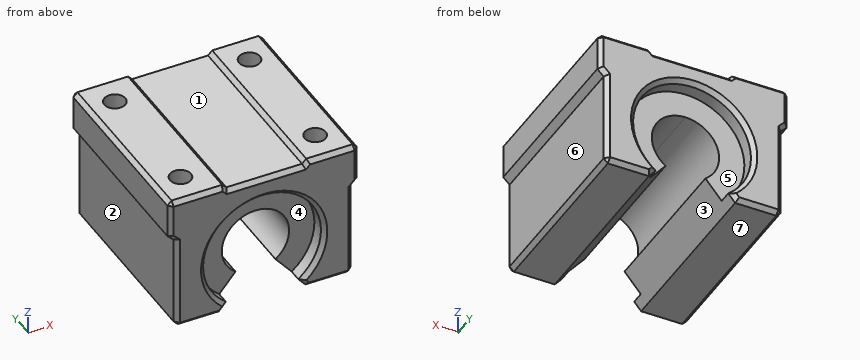
```python
from build123d import *

# Parameters (mm, degrees)
F1_DEPTH = 45
F2_R     = 14
F3_DEPTH = 4
F4_R     = 14
F5_DEPTH = 4
F6_R     = 2.5
F7_DEPTH = 12
F8_SIZE  = 1


with BuildPart() as f1:
    # F0 (on Front) → F1 (new body)
    with BuildSketch(Plane.XZ):
        with BuildLine():
            Line((13, 33), (0, 33))
            Line((0, 33), (0, 24))
            Line((0, 24), (1.5, 22.5))
            Line((1.5, 22.5), (1.5, 0))
            Line((1.5, 0), (12.250585, 0))
            Line((12.250585, 0), (17.754591, 6.559418))
            ThreePointArc((17.754591, 6.559418), (14.899847, 15.497533), (22.5, 21))
            ThreePointArc((22.5, 21), (30.100153, 15.497533), (27.245409, 6.559418))
            Line((27.245409, 6.559418), (32.749415, 0))
            Line((32.749415, 0), (43.5, 0))
            Line((43.5, 0), (43.5, 22.5))
            Line((43.5, 22.5), (45, 24))
            Line((45, 24), (45, 33))
            Line((45, 33), (33, 33))
            Line((33, 33), (32, 32))
            Line((32, 32), (14, 32))
            Line((14, 32), (13, 33))
        make_face()
    extrude(amount=F1_DEPTH)

    # F2 (on face) → F3 (cut)
    with BuildSketch(Plane.XZ.offset(45)):
        with Locations((22.5, 13)):
            Circle(F2_R)
    extrude(amount=-F3_DEPTH, mode=Mode.SUBTRACT)

    # F4 (on face) → F5 (cut)
    with BuildSketch(Plane(origin=(0, 0, 0), x_dir=(-1, 0, 0), z_dir=(0, 1, 0))):
        with Locations((-22.5, 13)):
            Circle(F4_R)
    extrude(amount=-F5_DEPTH, mode=Mode.SUBTRACT)

    # F6 (on face) → F7 (cut)
    with BuildSketch(Plane.XY.offset(33)):
        with Locations((6.5, -37.5)):
            Circle(F6_R)
        with Locations((38.5, -37.5)):
            Circle(F6_R)
        with Locations((6.5, -7.5)):
            Circle(F6_R)
        with Locations((38.5, -7.5)):
            Circle(F6_R)
    extrude(amount=-F7_DEPTH, mode=Mode.SUBTRACT)

    # F8
    f8_edges = [f1.edges().sort_by_distance(p)[0] for p in [
        (22.5, 0, 27),
        (31.927972, 0, 0.978957),
        (38.124707, 0, 0),
        (43.5, 0, 11.25),
        (44.25, 0, 23.25),
        (45, 0, 28.5),
        (39, 0, 33),
        (32.5, 0, 32.5),
        (23, 0, 32),
        (13.5, 0, 32.5),
        (6.5, 0, 33),
        (0, 0, 28.5),
        (0.75, 0, 23.25),
        (1.5, 0, 11.25),
        (6.875293, 0, 0),
        (13.072028, 0, 0.978957),
        (22.5, -45, 27),
        (31.927972, -45, 0.978957),
        (38.124707, -45, 0),
        (43.5, -45, 11.25),
        (44.25, -45, 23.25),
        (45, -45, 28.5),
        (39, -45, 33),
        (32.5, -45, 32.5),
        (23, -45, 32),
        (13.5, -45, 32.5),
        (6.5, -45, 33),
        (0, -45, 28.5),
        (0.75, -45, 23.25),
        (1.5, -45, 11.25),
        (6.875293, -45, 0),
        (13.072028, -45, 0.978957),
        (45, -22.5, 33),
        (0, -22.5, 33),
        (1.5, -22.5, 0),
        (43.5, -22.5, 0),
    ]]
    chamfer(f8_edges, length=F8_SIZE)


solid = f1.part
```
Source: CAD feature listing. Evaluate the final solid. Frame: model axes, mm. Face numbers are marked on the shaded views. A direction names the side the tool comes from. Give positions to 0.01 mm unless a question says otherwise; leave off trailing zeros. Loops run counter-clockwise (first coordinate to the right, second up) from the corner with the lowest first, then second, coordinate; pieces in that order, holes last. Notation, with made-up numbers: (8.25, 20) -> (61.25, 20) arc R20 cw to (61.25, 39) -> close; hole circle Ø9 at (89.25, 77.5). An arc over 180 degrees is marked (long way). Use a Markdown table: item, result. Add a question column.
(1) Section query C-C (x = 38.5). Output: boundary loops of the cut face in (y, z).
(2) Section query A-A (z = 13). Output: boundary loops of the cut face in (x, y).
(3) Section query B-B (y = -21). Output: boundary loops of the cut face in (x, z), then the cut area to 3 significant figures.
(4) Access query for the marked faces 1, 2, 3 and 4. Directions: +Z, -Z, +X, -X, +Y, -Y. A direction counts if a zero-diameter tool reaches every point of the face in a straight line with its end or side. Return the directions, or none.
(5) Pull-direction query (Z, two-part tool) for the marked faces 5, 6 and 7; classes: +Z half, -Z half, draft (parallel to the pull), parting line (faces both ways), or undercut.
(6) First-contact query: pin 1 Ø2.5 at (x, y) = (39.5, -37.5) entering from +Z; pin 2 Ø17 at (y, z) = (-26.5, 11.5) entering from -X; pin 3 Ø8 at (y, z) = (-26, 7) entering from +X. Flat tips, straight axial feed; report the tip coordinate or a pass-through.
(7) Ray query, line 1 (Y direction, x = 38.5, z = 29.5); line 2 (X direction, y = -41.8, z = 13); line 3 (X direction, y = -9, z = 24). Return the intervals inside material, ascending.
(8) Section query D-D (y = -7.5). Output: boundary loops of the cut face in (x, z), then the cut area to 3 significant figures.
Checked values:
| question | item | result |
|---|---|---|
| 1 | outline | (-45, 1) -> (-44, 0) -> (-1, 0) -> (0, 1) -> (0, 32) -> (-1, 33) -> (-5, 33) -> (-5, 21) -> (-10, 21) -> (-10, 33) -> (-35, 33) -> (-35, 21) -> (-40, 21) -> (-40, 33) -> (-44, 33) -> (-45, 32) -> close |
| 2 | outline | (1.5, -44) -> (2.5, -45) -> (7.5, -45) -> (8.5, -44) -> (8.5, -41) -> (14.5, -41) -> (14.5, -4) -> (8.5, -4) -> (8.5, -1) -> (7.5, 0) -> (2.5, 0) -> (1.5, -1) -> close; (30.5, -41) -> (36.5, -41) -> (36.5, -44) -> (37.5, -45) -> (42.5, -45) -> (43.5, -44) -> (43.5, -1) -> (42.5, 0) -> (37.5, 0) -> (36.5, -1) -> (36.5, -4) -> (30.5, -4) -> close |
| 3 | outline | (0, 24) -> (1.5, 22.5) -> (1.5, 1) -> (2.5, 0) -> (12.25, 0) -> (17.75, 6.56) arc R8 cw (long way) to (27.25, 6.56) -> (32.75, 0) -> (42.5, 0) -> (43.5, 1) -> (43.5, 22.5) -> (45, 24) -> (45, 32) -> (44, 33) -> (33, 33) -> (32, 32) -> (14, 32) -> (13, 33) -> (1, 33) -> (0, 32) -> close |
| 3 | area | 1,100 mm^2 |
| 4 | face 1 | +Z, +Y, -Y |
| 4 | face 2 | -Z, -X, +Y, -Y |
| 4 | face 3 | -Z, +Y, -Y |
| 4 | face 4 | -Y |
| 5 | face 5 | undercut |
| 5 | face 6 | draft |
| 5 | face 7 | -Z half |
| 6 | pin 1 | z = 21 |
| 6 | pin 2 | x = 1.5 |
| 6 | pin 3 | x = 43.5 |
| 7 | line 1 | -45 to -40, -35 to -10, -5 to 0 |
| 7 | line 2 | 1.5 to 8.5, 36.5 to 43.5 |
| 7 | line 3 | 0 to 4.5, 8.5 to 36.5, 40.5 to 45 |
| 8 | outline | (0, 24) -> (1.5, 22.5) -> (1.5, 1) -> (2.5, 0) -> (12.25, 0) -> (17.75, 6.56) arc R8 cw (long way) to (27.25, 6.56) -> (32.75, 0) -> (42.5, 0) -> (43.5, 1) -> (43.5, 22.5) -> (45, 24) -> (45, 32) -> (44, 33) -> (41, 33) -> (41, 21) -> (36, 21) -> (36, 33) -> (33, 33) -> (32, 32) -> (14, 32) -> (13, 33) -> (9, 33) -> (9, 21) -> (4, 21) -> (4, 33) -> (1, 33) -> (0, 32) -> close |
| 8 | area | 985 mm^2 |
